Geometry: final body of the model. Coordinates: model frame, mm. A direction names the side the tool comes from. Give positions to 0.01 mm unless a question says otherwise; leave off trailing zeros. Order: outer loops, then holes, each group sorted by start corner. A loop starts at its lowest first (then second) coordinate and runs counter-clockwise, first axis right, second up. Notation, with made-up numbers: (-8.5, 72.5) -> (2.5, 72.5) arc R19 cw to (2.5, 76.5) -> close; hole circle Ø4 at (41.25, 5.5). An arc over 180 degrees is marked (long way). Answer in a Markdown table with one row per item. Add a question column.
Q1. Cut plane B-B on x = 2.2. Return the cut outline in (y, z), and give its area (3 significant figures).
Q2. Cut plane D-D on z = -3.5. Return the cut outline in (x, y).
Q3. Cut plane A-A on z = 0. Return the cut outline in (x, y), and give its area (3 significant figures).
Q4. Cut plane C-C on y = -1. Return the cut outline in (x, z).
Q5. Set-up query: faces 1 (the face through (1.479, 1.233, -2.175)), 2 (the face through (0, 3, 0)). Return all of +Z, -Z, +X, -X, +Y, -Y with unobstructed straight access to the full face (end or side cutting, diameter ignored); none if empty.
Q6. Pull-direction query (Z, two-part tool) for faces 3 (the face through (1.479, 1.267, 2.155)), 4 (the face through (1.48, -5.37, 1.19)), 5 (the face through (3, 3, 0)); classes: +Z half, -Z half, draft (parallel to the pull), parting line (faces both ways), or undercut.
Q7. Line query: line 1 along Y through (x, z) = (2.05, 0); line 2 along Z through (x, y) = (0.8, -1.75); line 3 along Y through (x, z) = (1.55, -2.5). Output: solid intervals per line, ascending. Write a range as from..to.
from build123d import *

# Parameters (mm, degrees)
SKETCH_1_R      = 5.5
EXTRUDE_1_DEPTH = 3


with BuildPart() as part:
    # 草图1 → 凸台-拉伸1 (new body)
    with BuildSketch(Plane(origin=(0, 0, 0), x_dir=(0, 0, -1), z_dir=(1, 0, 0))):
        Circle(SKETCH_1_R)
        Polygon((2.886751346, 0), (1.443375673, 2.5), (-1.443375673, 2.5), (-2.886751346, 0), (-1.443375673, -2.5), (1.443375673, -2.5), align=None, mode=Mode.SUBTRACT)
    extrude(amount=EXTRUDE_1_DEPTH)


solid = part.part
Completed:
| question | item | result |
|---|---|---|
| 1 | outline | circle Ø11 at (0, 0); hole (-2.5, -1.44) -> (0, -2.89) -> (2.5, -1.44) -> (2.5, 1.44) -> (0, 2.89) -> (-2.5, 1.44) -> close |
| 1 | area | 73.4 mm² |
| 2 | outline | (0, -4.24) -> (3, -4.24) -> (3, 4.24) -> (0, 4.24) -> close |
| 3 | outline | (0, -5.5) -> (3, -5.5) -> (3, -2.5) -> (0, -2.5) -> close; (0, 2.5) -> (3, 2.5) -> (3, 5.5) -> (0, 5.5) -> close |
| 3 | area | 18.0 mm² |
| 4 | outline | (0, -5.41) -> (3, -5.41) -> (3, -2.31) -> (0, -2.31) -> close; (0, 2.31) -> (3, 2.31) -> (3, 5.41) -> (0, 5.41) -> close |
| 5 | face 1 | +X, -X |
| 5 | face 2 | +Z, -Z, -X, +Y, -Y |
| 6 | face 3 | undercut |
| 6 | face 4 | parting line |
| 6 | face 5 | draft |
| 7 | line 1 | y = -5.5..-2.5, 2.5..5.5 |
| 7 | line 2 | z = -5.21..-1.88, 1.88..5.21 |
| 7 | line 3 | y = -4.9..-0.67, 0.67..4.9 |
